from build123d import *

# Parameters (mm, degrees)
SKETCH1_W           = 45
SKETCH1_H           = 20
BOSS_EXTRUDE1_DEPTH = 3
SKETCH2_R           = 7.5
SKETCH2_R_2         = 6.5
BOSS_EXTRUDE2_DEPTH = 12
SKETCH2_2_R         = 6.5
BOSS_EXTRUDE3_DEPTH = 10
BOSS_EXTRUDE4_DEPTH = 2


with BuildPart() as part:
    # Sketch1 → Boss-Extrude1 (new body)
    with BuildSketch(Plane.XY):
        with Locations((22.5, 10)):
            Rectangle(SKETCH1_W, SKETCH1_H)
    extrude(amount=BOSS_EXTRUDE1_DEPTH)

    # Sketch2 → Boss-Extrude2 (add)
    # profile 1 of 2: a face of its own
    with BuildSketch(Plane.XY.offset(3)):
        with Locations(Location((10, 10, 0), (0, 0, 180))):
            Circle(SKETCH2_R)
        with Locations((10, 10)):
            Circle(SKETCH2_R_2, mode=Mode.SUBTRACT)
    # profile 2 of 2: a face of its own
    with BuildSketch(Plane.XY.offset(3)):
        with Locations(Location((35, 10, 0), (0, 0, 180))):
            Circle(SKETCH2_R)
        with Locations((35, 10)):
            Circle(SKETCH2_R_2, mode=Mode.SUBTRACT)
    extrude(amount=BOSS_EXTRUDE2_DEPTH)

    # Sketch2_2 → Boss-Extrude3 (add)
    with BuildSketch(Plane.XY.offset(3)):
        with Locations((10, 10)):
            Circle(SKETCH2_2_R)
        with Locations((35, 10)):
            Circle(SKETCH2_2_R)
    extrude(amount=BOSS_EXTRUDE3_DEPTH)

    # Sketch3 → Boss-Extrude4 (add)
    with BuildSketch(Plane.XY.offset(3)):
        with BuildLine():
            Line((17.5, 19), (27.5, 19))
            ThreePointArc((27.5, 19), (28.5, 18), (27.5, 17))
            Line((27.5, 17), (17.5, 17))
            ThreePointArc((17.5, 17), (16.5, 18), (17.5, 19))
        make_face()
    extrude(amount=BOSS_EXTRUDE4_DEPTH)


solid = part.part
Verification items for the finished model (mm, model axes). A direction names the side the tool comes from. Give positions to 0.01 mm unless a question says otherwise; leave off trailing zeros. Order: outer loops, then holes, each group sorted by start corner. A loop starts at its lowest first (then second) coordinate and runs counter-clockwise, first axis right, second up. Notation, with made-up numbers: M 62,66 L 108,66 A29 ccw 108,88 Z; hole C -28.5,2.25 d1. An arc over 180 degrees is marked long. Use one line per item in the form item = value. Start each with the question number.
Q1. Mould release check, pull along Y, two halves, no side actions. Record for faces 4 (the cylindrical face through (28.506, 10.286, 13.986)), 5 (the flat face through (23, 18, 5)), 6 (the flat face through (23, 17, 4)): +Y half, -Y half, draft (parallel to the pull), parting line (faces both ways), or undercut.
Q2. Section check C-C (x = 19.5). Enter the section's corners in (y, z).
Q3. Scan lines: line 1 along Y through (x, z) = (10, 14.35); line 2 along Z through (x, y) = (21.5, 10); line 3 along Z through (x, y) = (8, 9.75). Record each from-to range of solid material in increasing order. Write a range as [from, to].
Q4. Section check A-A (z = 4.5). Enter the section's corners in (x, y).
Q5. Go/stop test with flat-tipped pins: pin 1 Ø1 at (x, y) = (35.5, 12) entering from +Z; pin 2 Ø2 at (x, y) = (19.5, 3) entering from +Z; pin 3 Ø1 at (x, y) = (21, 18) entering from +Z. Record where each tip stops, or that it passes through.
Q6. Section check B-B (y = 18). Enter the section's corners in (x, z).
Q7. Access from +Z, -Z, +X, -X, +Y, -Y to the whole of each face (thin tool, end or side, straight path). Record for faces 1 (the flat face through (22, 0, 1)), 2 (the flat face through (10, 10, 13)), 3 (the flat face through (22, 19, 4)).
Q8. Section check D-D (z = 9.75). Enter the section's corners in (x, y), then the cut area to 3 significant figures.
Evaluation:
q1.face_4 = undercut
q1.face_5 = draft
q1.face_6 = -Y half
q2.outline = M 0,0 L 20,0 L 20,3 L 19,3 L 19,5 L 17,5 L 17,3 L 0,3 Z
q3.line_1 = [2.5, 3.5], [16.5, 17.5]
q3.line_2 = [0, 3]
q3.line_3 = [0, 13]
q4.outline = C 10,10 d15; M 17.5,17 L 27.5,17 A1 ccw 27.5,19 L 17.5,19 A1 ccw Z; C 35,10 d15
q5.pin_1 = 13
q5.pin_2 = 3
q5.pin_3 = 5
q6.outline = M 0,0 L 45,0 L 45,3 L 28.5,3 L 28.5,5 L 16.5,5 L 16.5,3 L 0,3 Z
q7.face_1 = +Z, -Z, +X, -X, -Y
q7.face_2 = +Z
q7.face_3 = +Z, +X, -X, +Y
q8.outline = C 10,10 d15; C 35,10 d15
q8.area = 353 mm2
